Build history of the part. All positions in model axes, mm. Round coordinates to 2 decimals unless told otherwise and drop trailing zeros.
from build123d import *

# Parameters (mm, degrees)
SKETCH1_W           = 200.025
SKETCH1_H           = 200.025
SKETCH1_R           = 5.08
SKETCH1_W_2         = 27.758924323
SKETCH1_H_2         = 15.850492031
SKETCH1_W_3         = 31.563171913
SKETCH1_H_3         = 7.913427648
BOSS_EXTRUDE1_DEPTH = 6.35
FILLET1_R           = 5.08
SKETCH3_R           = 2.4
CUT_EXTRUDE1_DEPTH  = 142.598203764
SKETCH4_W           = 200.025
SKETCH4_H           = 200.025
SKETCH4_R           = 5.08
SKETCH4_W_2         = 149.225
SKETCH4_H_2         = 149.17772653
SKETCH4_W_3         = 27.758924323
SKETCH4_H_3         = 15.850492031
SKETCH4_W_4         = 31.563171913
SKETCH4_H_4         = 7.913427648
BOSS_EXTRUDE2_DEPTH = 0.0254
SKETCH5_R           = 8.89
CUT_EXTRUDE2_DEPTH  = 142.598203764


with BuildPart() as part:
    # Sketch1 → Boss-Extrude1 (new body)
    with BuildSketch(Plane(origin=(0, 0, 0), x_dir=(1, 0, 0), z_dir=(0, 1, 0))):
        with Locations((0, -0.023636735)):
            Rectangle(SKETCH1_W, SKETCH1_H)
        with Locations(Location((-87.3125, 87.288863265, 0), (0, 0, 270))):
            Circle(SKETCH1_R, mode=Mode.SUBTRACT)
        with Locations(Location((87.3125, 87.288863265, 0), (0, 0, 90))):
            Circle(SKETCH1_R, mode=Mode.SUBTRACT)
        with Locations(Location((-87.3125, -87.288863265, 0), (0, 0, 90))):
            Circle(SKETCH1_R, mode=Mode.SUBTRACT)
        with Locations(Location((87.3125, -87.288863265, 0), (0, 0, 270))):
            Circle(SKETCH1_R, mode=Mode.SUBTRACT)
        with Locations((-19.766444167, 88.253617249)):
            Rectangle(SKETCH1_W_2, SKETCH1_H_2, mode=Mode.SUBTRACT)
        with Locations((23.505506165, 92.222149441)):
            Rectangle(SKETCH1_W_3, SKETCH1_H_3, mode=Mode.SUBTRACT)
        Polygon((54.27, -38.5), (54.27, 38.5), (54.293636735, 54.27), (38.5, 54.27), (-38.5, 54.27), (-54.27, 54.246363265), (-54.27, 38.5), (-54.27, -38.5), (-54.27, -54.293636735), (-42.77, -54.27), (-38.5, -54.27), (38.5, -54.27), (42.77, -54.27), (54.246363265, -54.27), (54.27, -42.77), align=None, mode=Mode.SUBTRACT)
    extrude(amount=BOSS_EXTRUDE1_DEPTH)

    # Fillet1
    fillet1_edges = [part.edges().sort_by_distance(p)[0] for p in [
        (-54.27, 3.175, -54.246363265),
        (-54.27, 3.175, 54.293636735),
        (54.246363265, 3.175, 54.27),
        (54.293636735, 3.175, -54.27),
    ]]
    fillet(fillet1_edges, radius=FILLET1_R)

    # Sketch3 → Cut-Extrude1 (cut, through all)
    with BuildSketch(Plane.XZ):
        with Locations(Location((-24, 65.5, 0), (0, 0, 270))):
            Circle(SKETCH3_R)
        with Locations(Location((24, 65.5, 0), (0, 0, 270))):
            Circle(SKETCH3_R)
        with Locations(Location((65.5, 24, 0), (0, 0, 270))):
            Circle(SKETCH3_R)
        with Locations(Location((65.5, -24, 0), (0, 0, 270))):
            Circle(SKETCH3_R)
        with Locations(Location((24, -65.5, 0), (0, 0, 270))):
            Circle(SKETCH3_R)
        with Locations(Location((-24, -65.5, 0), (0, 0, 270))):
            Circle(SKETCH3_R)
        with Locations(Location((-65.5, -24, 0), (0, 0, 270))):
            Circle(SKETCH3_R)
        with Locations(Location((-65.5, 24, 0), (0, 0, 270))):
            Circle(SKETCH3_R)
    extrude(amount=-CUT_EXTRUDE1_DEPTH, mode=Mode.SUBTRACT)

    # Sketch4 → Boss-Extrude2 (add)
    with BuildSketch(Plane(origin=(0, 6.35, 0), x_dir=(1, 0, 0), z_dir=(0, 1, 0))):
        with Locations((0, -0.023636735)):
            Rectangle(SKETCH4_W, SKETCH4_H)
        with Locations(Location((-87.3125, 87.288863265, 0), (0, 0, 270))):
            Circle(SKETCH4_R, mode=Mode.SUBTRACT)
        with Locations(Location((87.3125, 87.288863265, 0), (0, 0, 90))):
            Circle(SKETCH4_R, mode=Mode.SUBTRACT)
        with Locations(Location((87.3125, -87.288863265, 0), (0, 0, 270))):
            Circle(SKETCH4_R, mode=Mode.SUBTRACT)
        with Locations(Location((-87.3125, -87.288863265, 0), (0, 0, 90))):
            Circle(SKETCH4_R, mode=Mode.SUBTRACT)
        Rectangle(SKETCH4_W_2, SKETCH4_H_2, mode=Mode.SUBTRACT)
        with Locations((-19.766444167, 88.253617249)):
            Rectangle(SKETCH4_W_3, SKETCH4_H_3, mode=Mode.SUBTRACT)
        with Locations((23.505506165, 92.222149441)):
            Rectangle(SKETCH4_W_4, SKETCH4_H_4, mode=Mode.SUBTRACT)
    extrude(amount=BOSS_EXTRUDE2_DEPTH)

    # Sketch5 → Cut-Extrude2 (cut, through all)
    with BuildSketch(Plane(origin=(0, 6.35, 0), x_dir=(1, 0, 0), z_dir=(0, 1, 0))):
        with Locations(Location((-64.4525, 64.455022357, 0), (0, 0, 270))):
            Circle(SKETCH5_R)
        with Locations(Location((64.4525, 64.455022357, 0), (0, 0, 90))):
            Circle(SKETCH5_R)
    extrude(amount=-CUT_EXTRUDE2_DEPTH, mode=Mode.SUBTRACT)


solid = part.part
1) Slice it at A-A (x = -24). Count the separate pieces of the cut face and the enclosed holes in it, plus the area to 3 significant figures.
Results:
separate pieces: 5
enclosed holes: 0
area: 420 mm2
2) Mould opens along X. For faces 1 (the cylindrical face through (52.8, 3.22, 52.75)), 2 (the flat face through (-1, 6.35, 65)), 3 (the flat face through (100.012, 3, 1)) say: released by +X, released by -X, zero draft, split by the parting line, or undercut.
Results:
face 1: undercut
face 2: zero draft
face 3: released by +X
3) Pin check, flat tips, straight feed: pin 1 Ø7.5 at (x, z) = (24, 65.5) entering from -Y; pin 2 Ø6 at (x, z) = (-24, -65.5) entering from +Y. Stop position of each tip, or through.
Results:
pin 1: stops at y = 0
pin 2: stops at y = 6.35
4) Wall check: L1, parallel to X at y = 1.75, z = 65.5; L2, parallel to Z at x = -8, y = 1.75; L3, parallel to X at y = 4.5, z = 48. Give the ranges that are in metal, low to high.
Results:
L1: x = -100.01 to -26.4, -21.6 to 21.6, 26.4 to 100.01
L2: z = -99.99 to -96.18, -80.33 to -54.27, 54.27 to 100.04
L3: x = -100.01 to -54.27, 54.26 to 100.01
